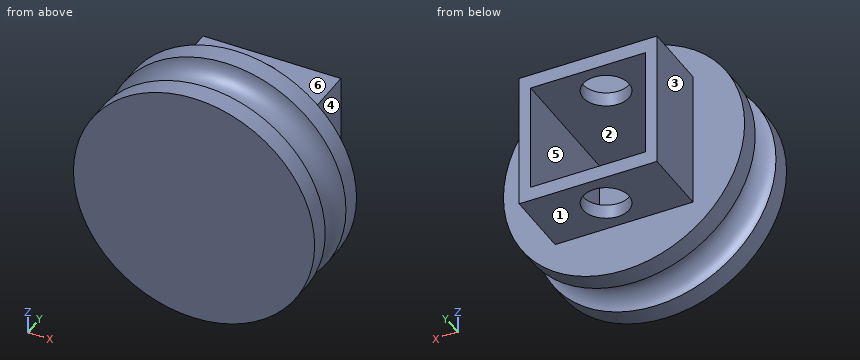
from build123d import *

# Parameters (mm, degrees)
CYLINDER019_R     = 10.5
CYLINDER019_DEPTH = 7
BOX016_W          = 12
BOX016_H          = 12
BOX016_DEPTH      = 6
BOX017_W          = 10
BOX017_H          = 9.5
BOX017_DEPTH      = 11.5
CYLINDER020_R     = 2
CYLINDER020_DEPTH = 12
TORUS_R           = 1.75


with BuildPart() as part:
    # Cylinder019 → Cylinder019 (join)
    with BuildSketch(Plane.XZ):
        Circle(CYLINDER019_R)
    extrude(amount=CYLINDER019_DEPTH)

    # Box016 → Box016 (join)
    with BuildSketch(Plane(origin=(-6, 0, 6), x_dir=(1, 0, 0), z_dir=(0, 1, 0))):
        with Locations((6, 6)):
            Rectangle(BOX016_W, BOX016_H)
    extrude(amount=BOX016_DEPTH)

    # Box017 → Box017 (cut)
    with BuildSketch(Plane(origin=(-5, 6, -4.75), x_dir=(1, 0, 0), z_dir=(0, -1, 0))):
        with Locations((5, 4.75)):
            Rectangle(BOX017_W, BOX017_H)
    extrude(amount=BOX017_DEPTH, mode=Mode.SUBTRACT)

    # Cylinder020 → Cylinder020 (cut)
    with BuildSketch(Plane(origin=(0, 3, 6), x_dir=(1, 0, 0), z_dir=(0, 0, -1))):
        Circle(CYLINDER020_R)
    extrude(amount=CYLINDER020_DEPTH, mode=Mode.SUBTRACT)

    # Torus → Torus (revolve, cut)
    with BuildSketch(Plane(origin=(0, -3.5, 0), x_dir=(1, 0, 0), z_dir=(0, 0, -1))):
        with Locations((10.75, 0)):
            Circle(TORUS_R)
    revolve(axis=Axis((0, -3.5, 0), (0, -1, 0)), mode=Mode.SUBTRACT)


with BuildPart() as part_1:
    # Body004 placement: moved
    add(part.part.moved(Location((0, -48, 0))))


solid = part_1.part
CAD build for the part. Positions are in the model's coordinates, mm. Face numbers are marked on the shaded views. A direction names the side the tool comes from. Give positions to 0.01 mm unless a question says otherwise; leave off trailing zeros. Write each loop counter-clockwise with the first axis right and the second up, starting at its lowest first coordinate (ties: lowest second). Pieces come first, ordered by that corner, then holes. Notation, with made-up numbers: (-23.75, 16) -> (11.25, 16) arc R16 ccw to (11.25, 36) -> close; hole circle Ø10 at (65, 73.5). An arc over 180 degrees is marked (long way). Return JSON: item names as keys, results as strings.
Item 1: Band-saw the part on C-C (z = 0). List the corners of the cut face in (x, y), then the cut area to 3 significant figures.
Answer below:
{"outline": "(-10.5, -55) -> (10.5, -55) -> (10.5, -53.23) arc R1.75 cw to (10.5, -49.77) -> (10.5, -48) -> (6, -48) -> (6, -42) -> (5, -42) -> (5, -53.5) -> (-5, -53.5) -> (-5, -42) -> (-6, -42) -> (-6, -48) -> (-10.5, -48) -> (-10.5, -49.77) arc R1.75 cw to (-10.5, -53.23) -> close", "area": "96.1 mm2"}
Item 2: Drill centre lines: probe 1 along X at (y, z) = (-45, 5.7); probe 2 along X at (y, z) = (-46, 0.75); probe 3 along Y at (x, z) = (0, 5.5). Where is each one in solid material? Low to high.
Answer below:
{"probe 1": "x = -6 to -2, 2 to 6", "probe 2": "x = -6 to -5, 5 to 6", "probe 3": "y = -55 to -47, -43 to -42"}
Item 3: Band-saw the part on D-D (y = -52.75). List the corners of the cut face in (x, z).
Answer below:
{"outline": "circle Ø19.05 at (0, 0); hole (-5, -4.75) -> (5, -4.75) -> (5, 4.75) -> (-5, 4.75) -> close"}
Item 4: Drop flat-ended pins along their axis: pin 1 (5 mm diameter, centred on x = -0.5, y = -45, fed in from +Z); pin 2 (3 mm diameter, centred on x = 3, y = -43.5, fed in from -Z); pin 3 (5 mm diameter, centred on y = -44, z = -1, fed in from -X); pin 4 (3.5 mm diameter, centred on x = 0, y = -45, fed in from +Z). Give the stop position or say it passes through.
Answer below:
{"pin 1": "stops at z = 6", "pin 2": "stops at z = -6", "pin 3": "stops at x = -6", "pin 4": "passes through"}
Item 5: Band-saw the part on B-B (y = -45). List the corners of the cut face in (x, z).
Answer below:
{"outline": "(-6, -6) -> (-2, -6) -> (-2, -4.75) -> (-5, -4.75) -> (-5, 4.75) -> (-2, 4.75) -> (-2, 6) -> (-6, 6) -> close; (2, -6) -> (6, -6) -> (6, 6) -> (2, 6) -> (2, 4.75) -> (5, 4.75) -> (5, -4.75) -> (2, -4.75) -> close"}
Item 6: Two-plate mould, pull along Z, no slides. Class the marked faces 4, 5 and 6: +Z half, -Z half, draft (parallel to the pull), parting line (faces both ways), or undercut.
Answer below:
{"face 4": "draft", "face 5": "undercut", "face 6": "+Z half"}
Item 7: Tool access for the marked faces 1, 2 and 3: list every direction of +Z, -Z, +X, -X, +Y, -Y with a clear straight run to the whole face (end or side of a thin tool).
Answer below:
{"face 1": "-Z, +X, -X, +Y", "face 2": "+Y", "face 3": "+Z, -Z, -X, +Y"}
Item 8: Band-saw the part on A-A (x = 0). List the corners of the cut face in (y, z), then the cut area to 3 significant figures.
Answer below:
{"outline": "(-55, -10.5) -> (-53.23, -10.5) arc R1.75 cw to (-49.77, -10.5) -> (-48, -10.5) -> (-48, -6) -> (-47, -6) -> (-47, -4.75) -> (-53.5, -4.75) -> (-53.5, 4.75) -> (-47, 4.75) -> (-47, 6) -> (-48, 6) -> (-48, 10.5) -> (-49.77, 10.5) arc R1.75 cw to (-53.23, 10.5) -> (-55, 10.5) -> close; (-43, -6) -> (-42, -6) -> (-42, -4.75) -> (-43, -4.75) -> close; (-43, 4.75) -> (-42, 4.75) -> (-42, 6) -> (-43, 6) -> close", "area": "91.9 mm2"}
